```python
from build123d import *

# Parameters (mm, degrees)
BOSS_EXTRUDE2_DEPTH      = 1.5
BOSS_EXTRUDE2_DEPTH_BACK = 1.5
SKETCH1_R                = 1.575
SKETCH1_R_2              = 2.05
SKETCH1_R_3              = 2.1
SKETCH1_R_4              = 1.6
SKETCH1_W                = 40.5
SKETCH1_H                = 20.499999995
SKETCH1_W_2              = 3.15
SKETCH1_H_2              = 3.15


with BuildPart() as part:
    # Sketch1 → Boss-Extrude2 (new, two sides: drawn at the far end of the back side and taken through both)
    with BuildSketch(Plane(origin=(0, 0, 0), x_dir=(0, 0, -1), z_dir=(1, 0, 0)).offset(-BOSS_EXTRUDE2_DEPTH_BACK)):
        Polygon((11.425, 0), (8.5, 0), (8.5, -3), (5.5, -3), (5.5, 0), (0, 0), (0, 197), (156, 197), (156, 0), (150.5, 0), (150.5, -3), (147.5, -3), (147.5, 0), (144.575, 0), (144.575, 6.5), (147, 6.5), (147, 9), (139, 9), (139, 6.5), (141.425, 6.5), (141.425, 0), (138.5, 0), (138.5, -3), (135.5, -3), (135.5, 0), (20.5, 0), (20.5, -3), (17.5, -3), (17.5, 0), (14.575, 0), (14.575, 6.5), (17, 6.5), (17, 9), (9, 9), (9, 6.5), (11.425, 6.5), align=None)
        with Locations((5.25, 25.575)):
            Circle(SKETCH1_R, mode=Mode.SUBTRACT)
        with Locations(Location((5.25, 171.425, 0), (0, 0, 180))):
            Circle(SKETCH1_R, mode=Mode.SUBTRACT)
        with Locations((150.75, 171.425)):
            Circle(SKETCH1_R, mode=Mode.SUBTRACT)
        with Locations(Location((150.75, 25.575, 0), (0, 0, 180))):
            Circle(SKETCH1_R, mode=Mode.SUBTRACT)
        with Locations((73.2, 5.35)):
            Circle(SKETCH1_R_2, mode=Mode.SUBTRACT)
        with Locations((73.2, 17.149999995)):
            Circle(SKETCH1_R_2, mode=Mode.SUBTRACT)
        with Locations((21.2, 5.35)):
            Circle(SKETCH1_R_2, mode=Mode.SUBTRACT)
        with Locations((21.2, 17.149999995)):
            Circle(SKETCH1_R_2, mode=Mode.SUBTRACT)
        with Locations((40.1, 75)):
            Circle(SKETCH1_R_3, mode=Mode.SUBTRACT)
        with Locations((40.1, 150.8)):
            Circle(SKETCH1_R_3, mode=Mode.SUBTRACT)
        with Locations(Location((115.9, 75, 0), (0, 0, 180))):
            Circle(SKETCH1_R_3, mode=Mode.SUBTRACT)
        with Locations(Location((115.9, 150.8, 0), (0, 0, 180))):
            Circle(SKETCH1_R_3, mode=Mode.SUBTRACT)
        with Locations((88, 182)):
            Circle(SKETCH1_R_4, mode=Mode.SUBTRACT)
        with Locations((68, 182)):
            Circle(SKETCH1_R_4, mode=Mode.SUBTRACT)
        with Locations((47.2, 11.249999997)):
            Rectangle(SKETCH1_W, SKETCH1_H, mode=Mode.SUBTRACT)
        with Locations((5.25, 17.575)):
            Rectangle(SKETCH1_W_2, SKETCH1_H_2, mode=Mode.SUBTRACT)
        with Locations((5.25, 33.575)):
            Rectangle(SKETCH1_W_2, SKETCH1_H_2, mode=Mode.SUBTRACT)
        with Locations((5.25, 163.425)):
            Rectangle(SKETCH1_W_2, SKETCH1_H_2, mode=Mode.SUBTRACT)
        with Locations((5.25, 179.425)):
            Rectangle(SKETCH1_W_2, SKETCH1_H_2, mode=Mode.SUBTRACT)
        with Locations((150.75, 179.425)):
            Rectangle(SKETCH1_W_2, SKETCH1_H_2, mode=Mode.SUBTRACT)
        with Locations((150.75, 163.425)):
            Rectangle(SKETCH1_W_2, SKETCH1_H_2, mode=Mode.SUBTRACT)
        with Locations((150.75, 33.575)):
            Rectangle(SKETCH1_W_2, SKETCH1_H_2, mode=Mode.SUBTRACT)
        with Locations((150.75, 17.575)):
            Rectangle(SKETCH1_W_2, SKETCH1_H_2, mode=Mode.SUBTRACT)
    extrude(amount=BOSS_EXTRUDE2_DEPTH + BOSS_EXTRUDE2_DEPTH_BACK)


solid = part.part
```
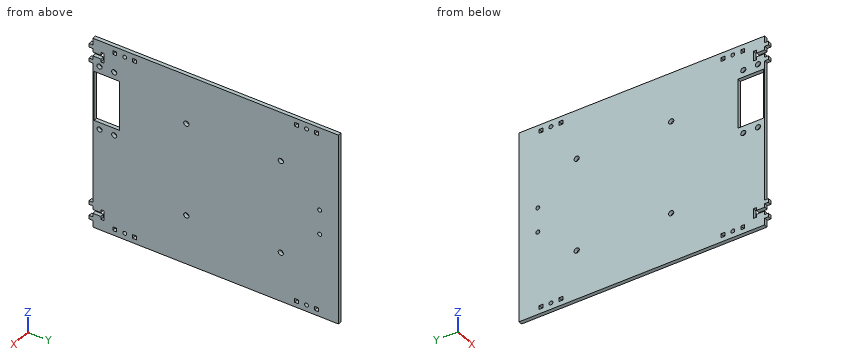
For this review, take the finished solid that the model builds, in its own axes (mm). Coordinates: 2 decimals unless noted, no trailing zeros. Write each loop counter-clockwise with the first axis right and the second up, starting at its lowest first coordinate (ties: lowest second). Pieces come first, ordered by that corner, then holes. Notation, with made-up numbers: (61.5, 30) -> (117.5, 30) arc R5 ccw to (117.5, 39) -> close; hole circle Ø8 at (36.5, 35.5). An arc over 180 degrees is marked (long way). Put each result on its own line as item: value.
Q1. Clearance check with flat-ended pins moving along their axes: pin 1 Ø0.9 at (x, y) = (0, -1.5) entering from -Z; pin 2 Ø0.9 at (x, z) = (0.5, -10.5) entering from -Y; pin 3 Ø0.9 at (x, y) = (0, -1.5) entering from +Z. State where each tip first meets the part, or that it passes through.
From the geometry:
pin 1: stops at z = -150.5
pin 2: stops at y = 0
pin 3: stops at z = -5.5
Q2. Take a section at B-B, the plane y = 75. State the section outline as (x, z) points.
From the geometry:
outline: (-1.5, -156) -> (1.5, -156) -> (1.5, -118) -> (-1.5, -118) -> close; (-1.5, -113.8) -> (1.5, -113.8) -> (1.5, -42.2) -> (-1.5, -42.2) -> close; (-1.5, -38) -> (1.5, -38) -> (1.5, 0) -> (-1.5, 0) -> close
Q3. Take a section at A-A, the plane z = -30.5. State the section outline as (x, y) points, then the cut area to 4 significant figures.
From the geometry:
outline: (-1.5, 0) -> (1.5, 0) -> (1.5, 1) -> (-1.5, 1) -> close; (-1.5, 21.5) -> (1.5, 21.5) -> (1.5, 197) -> (-1.5, 197) -> close
area: 529.5 mm2
Q4. Take a section at C-C, the plane x = 0.65. Count the separate pieces of the cut face and the enclosed holes in it, then the cut area to 3 significant figures.
From the geometry:
separate pieces: 1
enclosed holes: 23
area: 29,600 mm2
Q5. Wall thickness on L1, parallel to Y at x = -0.5, z = -73.2; L2, parallel to Y at x = -0.35, z = -115.9; L3, parallel to Z at x = -0.3, y = 178.5 (3 decimals): over which ranges is each line inside the solid? List them lowest first.
From the geometry:
L1: y = 0 to 3.3, 7.4 to 15.1, 19.2 to 197
L2: y = 0 to 72.9, 77.1 to 148.7, 152.9 to 197
L3: z = -156 to -152.325, -149.175 to -6.825, -3.675 to 0
